Input: part model. Units: mm. Frame: model coordinates. Round coordinates to 2 decimals unless told otherwise and drop trailing zeros. Write each loop counter-clockwise with the first axis right and the second up, starting at its lowest first coordinate (ties: lowest second). Pieces come first, ordered by that corner, then holes. Notation, with made-up numbers: (-6, 81.5) - (1, 81.5) arc R6 cw to (1, 91.5) - close; hole circle Ø9 at (88, 65). An arc over 180 degrees is marked (long way). One line per item, written item: value. Start each with the question number.
```python
from build123d import *

# Parameters (mm, degrees)
SKETCH1_W           = 36.0426
SKETCH1_H           = 21.7424
BOSS_EXTRUDE1_DEPTH = 7.2136
SKETCH2_R           = 1.3462
CUT_EXTRUDE1_DEPTH  = 7.2136
FILLET1_R           = 2.032


with BuildPart() as part:
    # Sketch1 → Boss-Extrude1 (new body)
    with BuildSketch(Plane(origin=(0, 0, 0), x_dir=(1, 0, 0), z_dir=(0, 1, 0))):
        with Locations((-73.427135669, 1.514506775)):
            Rectangle(SKETCH1_W, SKETCH1_H)
    extrude(amount=BOSS_EXTRUDE1_DEPTH)

    # Sketch2 → Cut-Extrude1 (cut)
    with BuildSketch(Plane(origin=(0, 7.2136, 0), x_dir=(1, 0, 0), z_dir=(0, 1, 0))):
        with Locations((-57.907735669, 9.718706775)):
            Circle(SKETCH2_R)
        with Locations((-89.086235669, 8.118506775)):
            Circle(SKETCH2_R)
        with Locations((-57.907735669, -6.689693225)):
            Circle(SKETCH2_R)
        with Locations((-89.086235669, -5.089493225)):
            Circle(SKETCH2_R)
    extrude(amount=-CUT_EXTRUDE1_DEPTH, mode=Mode.SUBTRACT)

    # Fillet1
    fillet1_edges = [part.edges().sort_by_distance(p)[0] for p in [
        (-91.448435669, 3.6068, -12.385706775),
        (-55.405835669, 3.6068, -12.385706775),
        (-55.405835669, 3.6068, 9.356693225),
        (-91.448435669, 3.6068, 9.356693225),
    ]]
    fillet(fillet1_edges, radius=FILLET1_R)


solid = part.part
```
Q1. Material intervals for probe 1 along X at (y, z) = (6, -9.75); probe 2 along Z at (x, y) = (-90, 4.75); probe 3 along X at (y, z) = (5.5, 4), sorted ascending. Write a range as from..to.
Q2. Cut plane A-A, the plane y = 3. Output: boundary loops of the cut face in (x, z).
Q3. Pull-direction query (Z, two-part tool) for faces 1 (the cylindrical face through (-56.02, 3.66, 8.78)), 2 (the flat face through (-55.406, 4, -1)), 3 (the cylindrical face through (-59.253, 3.657, -9.778)), 4 (the cylindrical face through (-59.253, 3.657, 6.631)); classes: pulls with the +Z half, pulls with the -Z half, needs draft (parallel to the pull), parting line crosses it, or undercut.
A:
1. probe 1: x = -91.45..-59.25, -56.56..-55.41
1. probe 2: z = -12.3..-9.11, -7.13..4.1, 6.08..9.27
1. probe 3: x = -91.45..-89.88, -88.3..-55.41
2. outline: (-91.45, -10.35) arc R2.03 ccw to (-89.42, -12.39) - (-57.44, -12.39) arc R2.03 ccw to (-55.41, -10.35) - (-55.41, 7.32) arc R2.03 ccw to (-57.44, 9.36) - (-89.42, 9.36) arc R2.03 ccw to (-91.45, 7.32) - close; hole circle Ø2.69 at (-89.09, -8.12); hole circle Ø2.69 at (-89.09, 5.09); hole circle Ø2.69 at (-57.91, -9.72); hole circle Ø2.69 at (-57.91, 6.69)
3. face 1: pulls with the +Z half
3. face 2: needs draft
3. face 3: undercut
3. face 4: undercut
